Verification items for this drawing (mm, ordinates from the low corner). A direction names the side the tool comes from. Coordinates: 2 decimals unless noted, no trailing zeros. Order: outer loops, then holes, each group sorted by start corner. A loop starts at its lowest first (then second) coordinate and runs counter-clockwise, first axis right, second up. Notation, with made-up numbers: (13, 36) - (62, 36) arc R38 ccw to (62, 75) - close; hole circle Ø3 at (2.5, 71.5). An arc over 180 degrees is marked (long way). Use CSV: the item, a comma, the result in double quotes. Start each with the question number.
1) Sectioned sample at B-B, the plane z = 3.25. Record the cut outline in (x, y), and give its area (3 significant figures).
2) Tool access check on the marked faces 1, 2, 3 and 4. Record the directions out of +Z, -Z, +X, -X, +Y, -Y that give a thin tool (end or side, any length) a straight path to the whole face; none if there is none.
3) Sectioned sample at C-C, the plane x = 54.5. Record the cut outline in (y, z).
4) Thickness scan on probe 1 along Y at (x, z) = (49.5, 16); probe 2 along X at (y, z) = (21, 6.75); probe 3 along Z at (x, y) = (17.5, 32.5). Record the ranges inside material, lowest first. Write a range as [from, to].
5) Sectioned sample at A-A, the plane y = 32. Record the cut outline in (x, z), and give its area (3 significant figures).
6) Depth check by flat-ended pin: P1, Ø3, axis at x = 28.5, y = 19.5, coming from the +Z side; P2, Ø4.5, axis at y = 23, z = 4.5, coming from the +X side; P3, Ø1, axis at x = 38.5, z = 9.5, coming from the -Y side. Enter the tip coordinate at first touch or a pass-through.
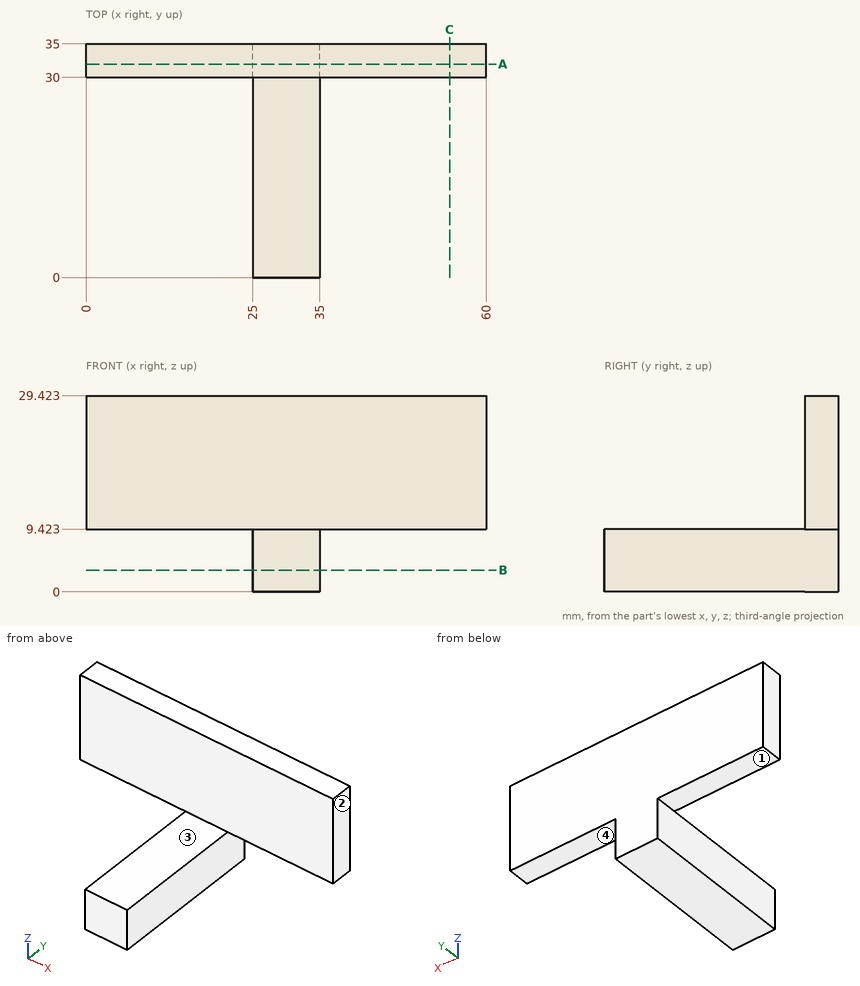
Evaluation:
1,outline,"(25, 0) - (35, 0) - (35, 35) - (25, 35) - close"
1,area,"350 mm²"
2,face 1,"-Z, -X, +Y, -Y"
2,face 2,"+Z, -Z, +X, +Y, -Y"
2,face 3,"+Z, +X, -X, -Y"
2,face 4,"-Z, +X, +Y, -Y"
3,outline,"(30, 9.42) - (35, 9.42) - (35, 29.42) - (30, 29.42) - close"
4,probe 1,"[30, 35]"
4,probe 2,"[25, 35]"
4,probe 3,"[9.42, 29.42]"
5,outline,"(0, 9.42) - (25, 9.42) - (25, 0) - (35, 0) - (35, 9.42) - (60, 9.42) - (60, 29.42) - (0, 29.42) - close"
5,area,"1,290 mm²"
6,P1,"z = 9.42"
6,P2,"x = 35"
6,P3,"y = 30"
